For this review, take the finished solid that the model builds, in its own axes (mm). A direction names the side the tool comes from. Give positions to 0.01 mm unless a question says otherwise; leave off trailing zeros. Order: outer loops, then holes, each group sorted by start corner. A loop starts at its lowest first (then second) coordinate and runs counter-clockwise, first axis right, second up. Notation, with made-up numbers: M -27.5,68.5 L -7.5,68.5 A37 cw -7.5,107.5 Z; hole C 40,-29.5 d4. An arc over 180 degrees is marked long. Answer as CSV lines item,"result". Start each with the question number.
1. We need section C-C, the plane y = -193.5. Give the boundary of the cut face in (x, z), and give its area (3 significant figures).
2. Mouldability with a two-part tool opening along X and no side actions: class faces 1 (the flat face through (-219.954, -175.987, 14.51)), 2 (the flat face through (-141, -131, 50)), 3 (the cylindrical face through (-371.063, -287.814, 25.264)) as pulls with the +X half, pulls with the -X half, needs draft (parallel to the pull), parting line crosses it, or undercut.
3. We need section A-A, the plane z = -8.5. Give the boundary of the cut face in (x, y), and give its area (3 significant figures).
4. Machinability: for faces 4 (the cylindrical face through (-371.063, 287.814, 25.264)), 5 (the flat face through (-219.954, 175.987, 14.51)), which of the approach directions +Z, -Z, +X, -X, +Y, -Y give a long, thin tool a straight path to every point of the face, cutting with its end or side? Answer none if there is none.
5. We need section B-B, the plane x = -139.5. Give the boundary of the cut face in (y, z), and give its area (3 significant figures).
6. Clearance check with flat-ended pins moving along their axes: P1, Ø5, axis at y = 261, z = 1, coming from the +X side; P2, Ø6, axis at y = -27.5, z = 31, coming from the +X side; P3, Ø10, axis at y = 24, z = -9.5, coming from the -X side. State where each tip first meets the part, or that it passes through.
7. For line 1 along Y through (x, z) = (-302.5, -15); line 2 along Y through (x, z) = (-91, 38); line 3 along X through (y, z) = (191.5, 43), list the stretches that pass through material, from the lowest coordinate up.
from build123d import *

# Parameters (mm, degrees)
PAD002_DEPTH           = 70
SKETCH006_R            = 6
POCKET002_DEPTH        = 30
SKETCH007_R            = 6
POCKET003_DEPTH        = 284.764355719
LINEARPATTERN001_COUNT = 4
LINEARPATTERN001_PITCH = 173.3333333333


with BuildPart() as part:
    # Sketch004 → Pad002 (new body)
    with BuildSketch(Plane.XY):
        with BuildLine():
            Line((-451.0352920823, 350), (16.0601402178, 22.9362572401))
            ThreePointArc((28, 0), (24.836303329, 12.9289611706), (16.0601402178, 22.9362572401))
            Line((18, 0), (28, 0))
            ThreePointArc((18, 0), (15.9661949972, 8.3114750382), (10.3243758543, 14.7447367972))
            Line((10.3243758543, 14.7447367972), (-456.7710564459, 341.8084795571))
            Line((-456.7710564459, 341.8084795571), (-451.0352920823, 350))
        make_face()
    extrude(amount=PAD002_DEPTH)

    # Sketch006 → Pocket002 (cut)
    with BuildSketch(Plane(origin=(0, 126.75, 0), x_dir=(-1, 0, 0), z_dir=(0, 1, 0))):
        with Locations((26.7405688034, 25.24131)):
            Circle(SKETCH006_R)
    extrude(amount=-POCKET002_DEPTH, mode=Mode.SUBTRACT)

    # Sketch007 (on Face2 of Pocket002) → Pocket003 (cut, through all)
    with BuildSketch(Plane(origin=(10.3243758543, 14.7447367972, 0), x_dir=(0.8191520443, -0.5735764364, 0), z_dir=(-0.5735764364, -0.8191520443, 0))):
        with Locations((-463.0458944975, 45)):
            Circle(SKETCH007_R)
    pocket003 = extrude(amount=-POCKET003_DEPTH, mode=Mode.SUBTRACT)

    # LinearPattern001: Pocket003 ×4
    with Locations(*[Vector(-0.8191520443, 0.5735764364, 0) * (i * LINEARPATTERN001_PITCH) for i in range(1, LINEARPATTERN001_COUNT)]):
        add(pocket003, mode=Mode.SUBTRACT)

    # Mirrored001: part across XZ


with BuildPart() as part_1:
    add(part.part)
    add(part.part.mirror(Plane.XZ))


with BuildPart() as part_2:
    # Body001 placement: moved
    add(part_1.part.moved(Location((0, 0, -20))))


solid = part_2.part
Result set:
1,outline,"M -244.96,-20 L -227.53,-20 L -227.53,50 L -244.96,50 Z"
1,area,"1,220 mm2"
2,face 1,"pulls with the -X half"
2,face 2,"needs draft"
2,face 3,"undercut"
3,outline,"M -456.77,-341.81 L -451.04,-350 L 16.06,-22.94 A28 ccw 16.06,22.94 L -451.04,350 L -456.77,341.81 L 10.32,14.74 A18 cw 10.32,-14.74 Z"
3,area,"11,800 mm2"
4,face 4,"none"
4,face 5,"+Z, -Z, -X"
5,outline,"M -131.86,-20 L -119.65,-20 L -119.65,50 L -131.86,50 Z; M 119.65,-20 L 131.86,-20 L 131.86,50 L 119.65,50 Z"
5,area,"1,710 mm2"
6,P1,"x = -320.36"
6,P2,"x = 13.83"
6,P3,"x = -10.03"
7,line 1,"-245.99 to -233.79, 233.79 to 245.99"
7,line 2,"-97.9 to -85.69, 85.69 to 97.9"
7,line 3,"-242.11 to -224.67"
